Geometry: final body of the model. Coordinates: model frame, mm. A direction names the side the tool comes from. Round coordinates to 2 decimals unless told otherwise and drop trailing zeros. Write each loop counter-clockwise with the first axis right and the second up, starting at its lowest first coordinate (ties: lowest second). Pieces come first, ordered by that corner, then holes. Notation, with made-up numbers: (-9, 72) -> (20, 72) arc R25 ccw to (20, 95) -> close; hole circle Ø5 at (12.25, 24.25). An arc over 180 degrees is marked (long way). Use one line per item in the form item = value. Start each with the question number.
1. Pin query (flat end, axial travel): pin 1 Ø10 at (x, y) = (-36.5, -11) entering from +Z; pin 2 Ø3 at (x, z) = (-58, 7.5) entering from +Y. Return the tip coordinate at first contact, or that it passes through.
2. Cut plane C-C, the plane z = 8. State how many separate pieces and enclosed holes the cut face has, plus the area to 3 significant figures.
3. Cut plane A-A, the plane y = -5. Return the cut outline in (x, z).
4. Line query: L1, parallel to X at y = 3, z = 2.5; L2, parallel to X at y = 32.5, z = 3.75; L3, parallel to Y at x = -59.5, z = 11. Output: solid intervals per line, ascending.
5. Cut plane D-D, the plane x = 3.5. Return the cut outline in (y, z), plus the area to 3 significant figures.
6. Draft query along Y for faces 1 (the face through (-1, -41, 1)), 2 (the face through (32.5, 0, 1)), 3 (the face through (60, -33, 3)), 4 (the face through (-61.8, 23, 5.7)). Return one class per face: pulls with the +Y half, pulls with the -Y half, needs draft (parallel to the pull), parting line crosses it, or undercut.
7. Cut plane B-B, the plane x = 60. Return the cut outline in (y, z).
8. Reachability of faces 5 (the face through (55, 30, 6)), 6 (the face through (-1, 1, 3)), 7 (the face through (-55, -30, 6)), 8 (the face through (52.5, -28, 7)) from +Z, -Z, +X, -X, +Y, -Y: full face, straight path, thin tool, end or side. Return the list, or none.
```python
from build123d import *

# Parameters (mm, degrees)
F0_W      = 135
F0_H      = 82
F1_DEPTH  = 3
F2_W      = 3
F2_H      = 10
F3_DEPTH  = 15
F4_DEPTH  = 15
F5_W      = 10
F5_H      = 15
F6_DEPTH  = 25
F8_D      = 5.5
F8_DEPTH  = 10
F8_TIP    = 1.6523667023
F12_COUNT = 2


# Not quite as in the source:
# - a feature names something its author has since deleted; it is built from what else it names


with BuildPart() as f1:
    # F0 (on Top) → F1 (new body)
    with BuildSketch(Plane.XY):
        Rectangle(F0_W, F0_H)
        with BuildLine():
            Line((-32.5, -32.5), (-32.5, 32.5))
            ThreePointArc((-32.5, 32.5), (-31.767766953, 34.267766953), (-30, 35))
            ThreePointArc((-30, 35), (-28.232233047, 34.267766953), (-27.5, 32.5))
            Line((-27.5, 32.5), (-27.5, -32.5))
            ThreePointArc((-27.5, -32.5), (-28.232233047, -34.267766953), (-30, -35))
            ThreePointArc((-30, -35), (-31.767766953, -34.267766953), (-32.5, -32.5))
        make_face(mode=Mode.SUBTRACT)
        with BuildLine():
            Line((27.5, -32.5), (27.5, 32.5))
            ThreePointArc((27.5, 32.5), (28.232233047, 34.267766953), (30, 35))
            ThreePointArc((30, 35), (31.767766953, 34.267766953), (32.5, 32.5))
            Line((32.5, 32.5), (32.5, -32.5))
            ThreePointArc((32.5, -32.5), (31.767766953, -34.267766953), (30, -35))
            ThreePointArc((30, -35), (28.232233047, -34.267766953), (27.5, -32.5))
        make_face(mode=Mode.SUBTRACT)
    extrude(amount=F1_DEPTH)

    # F2 (on face) → F3 (join)
    with BuildSketch(Plane.YZ.offset(67.5)):
        with Locations((-24.5, 8)):
            Rectangle(F2_W, F2_H)
    extrude(amount=-F3_DEPTH)

    # F2 (on face) → F4 (join)
    with BuildSketch(Plane.YZ.offset(67.5)):
        Polygon((-41, 3), (-26, 3), (-26, 13), align=None)
    extrude(amount=-F4_DEPTH)

    # F5 (on face) → F6 (cut)
    with BuildSketch(Plane.XY.offset(3)):
        with Locations((60, -33.5)):
            Rectangle(F5_W, F5_H)
    extrude(amount=F6_DEPTH, mode=Mode.SUBTRACT)

    # F8
    with Locations(Plane(origin=(0, -23, 0), x_dir=(-1, 0, 0), z_dir=(0, 1, 0))):
        with Locations((-60, 8)):
            Hole(F8_D / 2, depth=F8_DEPTH)
            with Locations((0, 0, -(F8_DEPTH + F8_TIP / 2))):  # 118° drill point
                Cone(0, F8_D / 2, F8_TIP, mode=Mode.SUBTRACT)

    # F10: F1 across plane


with BuildPart() as f1_1:
    add(f1.part)
    add(f1.part.mirror(Plane.YZ))

    # F12: F1 ×2 about axis
    f12_axis = Axis((0, 0, 10.3634241968), (0, 0, -1))


with BuildPart() as f1_2:
    add(f1_1.part)
    for i in range(1, F12_COUNT):
        add(f1_1.part.rotate(f12_axis, i * 360 / F12_COUNT))


solid = f1_2.part
```
Outcome:
q1.pin_1 = 3
q1.pin_2 = 26
q2.separate_pieces = 8
q2.enclosed_holes = 0
q2.area = 264 mm^2
q3.outline = (-67.5, 0) -> (-32.5, 0) -> (-32.5, 3) -> (-67.5, 3) -> close; (-27.5, 0) -> (27.5, 0) -> (27.5, 3) -> (-27.5, 3) -> close; (32.5, 0) -> (67.5, 0) -> (67.5, 3) -> (32.5, 3) -> close
q4.L1 = -67.5 to -32.5, -27.5 to 27.5, 32.5 to 67.5
q4.L2 = -67.5 to -65, -55 to -52.5, 52.5 to 55, 65 to 67.5
q4.L3 = -26 to -23, 23 to 26
q5.outline = (-41, 0) -> (41, 0) -> (41, 3) -> (-41, 3) -> close
q5.area = 246 mm^2
q6.face_1 = pulls with the -Y half
q6.face_2 = undercut
q6.face_3 = needs draft
q6.face_4 = undercut
q7.outline = (-41, 0) -> (41, 0) -> (41, 3) -> (26, 3) -> (26, 5.25) -> (23, 5.25) -> (23, 3) -> (-23, 3) -> (-23, 5.25) -> (-26, 5.25) -> (-26, 3) -> (-41, 3) -> close; (-26, 10.75) -> (-23, 10.75) -> (-23, 13) -> (-26, 13) -> close; (23, 10.75) -> (26, 10.75) -> (26, 13) -> (23, 13) -> close
q8.face_5 = +Z, +Y
q8.face_6 = +Z
q8.face_7 = +Z, -Y
q8.face_8 = +Z, +Y, -Y
